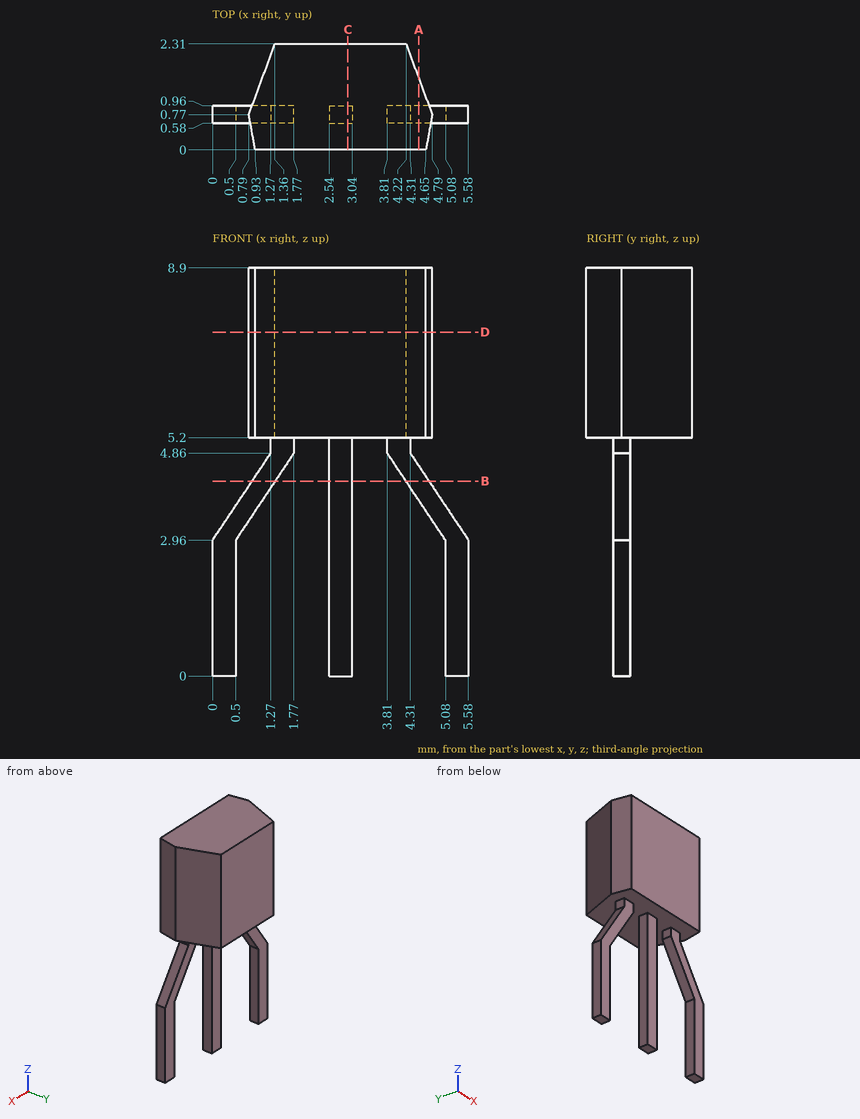
Here's the drawing with two shaded views (mm, measured from the low corner). I have some questions. Give positions to 0.01 mm unless a question says otherwise; leave off trailing zeros. Loops run counter-clockwise (first coordinate to the right, second up) from the corner with the lowest first, then second, coordinate; pieces in that order, holes last. Notation, with made-up numbers: (1, 68.25) -> (8, 68.25) arc R28 ccw to (8, 90.25) -> close; hole circle Ø1 at (76, 22.5). An arc over 180 degrees is marked (long way). Answer as a JSON object with one key per item and string values. Group by question number.
Item 1: Imagine slicing it at A-A on x = 4.5. Write out the boundary of the cut face in (y, z), then the cut area to 3 significant figures.
Item 2: Imagine slicing it at D-D on z = 7.5. Write out the boundary of the cut face in (x, y).
Item 3: Imagine slicing it at C-C on x = 2.95. Write out the boundary of the cut face in (y, z), then the cut area to 3 significant figures.
Item 4: Imagine slicing it at B-B on z = 4.25. Write out the boundary of the cut face in (x, y).
Item 5: Will these pins go through, and if not, where does the flat tip stop? pin 1 (1.5 mm diameter, centred on x = 3, z = 3, fed in from -Y); pin 2 (1.9 mm diameter, centred on x = 4.5, z = 3, fed in from +Y).
Item 6: I need wall thicknesses on L1, parallel to Z at x = 1.9, y = 1.8; L2, parallel to Z at x = 3.9, y = 0.85; L3, parallel to X at y = 0.55, z = 7.5. Which ranges of each line are inside material? Lowest first, please.
Answer list:
{
 "1": {"outline": "(0, 5.2) -> (1.55, 5.2) -> (1.55, 8.9) -> (0, 8.9) -> close; (0.58, 3.83) -> (0.96, 3.83) -> (0.96, 4.58) -> (0.58, 4.58) -> close", "area": "6.03 mm2"},
 "2": {"outline": "(0.79, 0.77) -> (0.93, 0) -> (4.65, 0) -> (4.79, 0.77) -> (4.22, 2.31) -> (1.36, 2.31) -> close"},
 "3": {"outline": "(0, 5.2) -> (0.58, 5.2) -> (0.58, 0) -> (0.96, 0) -> (0.96, 5.2) -> (2.31, 5.2) -> (2.31, 8.9) -> (0, 8.9) -> close", "area": "10.5 mm2"},
 "4": {"outline": "(0.86, 0.58) -> (1.36, 0.58) -> (1.36, 0.96) -> (0.86, 0.96) -> close; (2.54, 0.58) -> (3.04, 0.58) -> (3.04, 0.96) -> (2.54, 0.96) -> close; (4.22, 0.58) -> (4.72, 0.58) -> (4.72, 0.96) -> (4.22, 0.96) -> close"},
 "5": {"pin 1": "stops at y = 0.58", "pin 2": "stops at y = 0.96"},
 "6": {"L1": "z = 5.2 to 8.9", "L2": "z = 4.73 to 8.9", "L3": "x = 0.83 to 4.75"}
}
